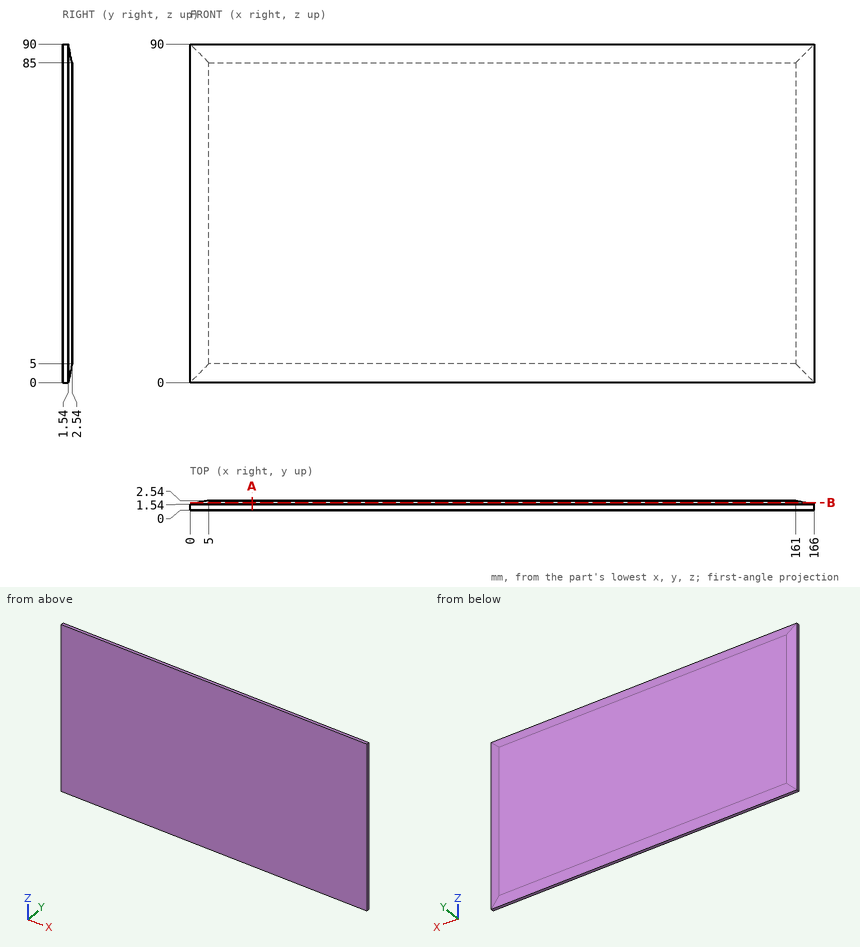
Here's the drawing with two shaded views (mm, measured from the low corner). I have some questions. Coordinates: 2 decimals unless noted, no trailing zeros. Order: outer loops, then holes, each group sorted by start corner. A loop starts at its lowest first (then second) coordinate and runs counter-clockwise, first axis right, second up. Notation, with made-up numbers: (74.25, -29.75) - (95.25, -29.75) arc R22 cw to (95.25, -0.75) - close; hole circle Ø10 at (52, 35). An arc over 180 degrees is marked (long way). Use CSV: the item, a comma, the result in double quotes. Start each with the question number.
1. I'm going to push a flat-ended pin straight in: pin 1 (4 mm diameter, centred on x = 68, z = 58.5, fed in from -Y). Where does the tip first touch, or does it pass through?
2. Suppose I cut it at A-A on x = 16.5. List the corners of the cut face in (y, z) for me.
3. Suppose I cut it at B-B on y = 2. List the corners of the cut face in (x, z) for me, then the cut area to 3 significant figures.
4. Please list where this line runs through material, in increasing order: line 1 (Y direction, x = 49, z = 4). Write a range as from..to.
Output:
1,pin 1,"stops at y = 0"
2,outline,"(0, 0) - (1.54, 0) - (2.54, 5) - (2.54, 85) - (1.54, 90) - (0, 90) - close"
3,outline,"(2.3, 2.3) - (163.7, 2.3) - (163.7, 87.7) - (2.3, 87.7) - close"
3,area,"13,800 mm2"
4,line 1,"y = 0..2.34"
